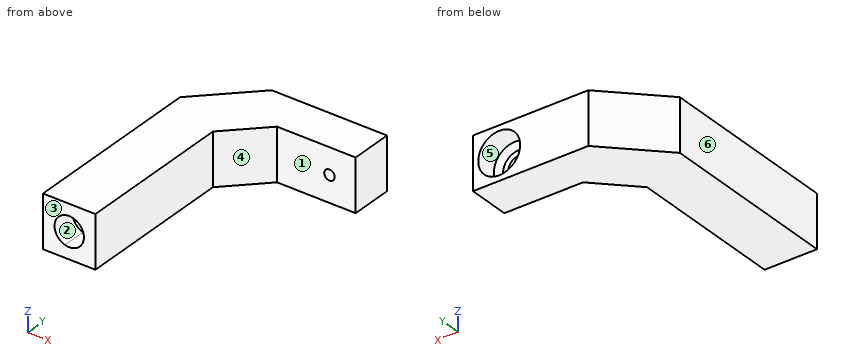
from build123d import *

# Parameters (mm, degrees)
PAD_DEPTH       = 10
CHAMFER_SIZE    = 10
POCKET_DEPTH    = 10.6
SKETCH002_R     = 2.8
POCKET001_DEPTH = 4.6
SKETCH003_R     = 1
POCKET002_DEPTH = 45.001
SKETCH004_R     = 4
POCKET003_DEPTH = 5
CHAMFER001_SIZE = 1
CHAMFER002_SIZE = 1


with BuildPart() as part:
    # Sketch → Pad (new body)
    with BuildSketch(Plane.XY):
        Polygon((22, 15), (-10, 15), (-10, -30), (0, -30), (0, 0), (7, 7), (22, 7), align=None)
    extrude(amount=PAD_DEPTH)

    # Chamfer
    chamfer_edges = [part.edges().sort_by_distance(p)[0] for p in [
        (-10, 15, 5),
    ]]
    chamfer(chamfer_edges, length=CHAMFER_SIZE)

    # Sketch001 → Pocket (cut)
    with BuildSketch(Plane.XZ.offset(30)):
        with BuildLine():
            ThreePointArc((-5.8, 2.316718), (-2.2, 5), (-5.8, 7.683282))
            Line((-5.8, 7.683282), (-5.8, 2.316718))
        make_face()
    extrude(amount=-POCKET_DEPTH, mode=Mode.SUBTRACT)

    # Sketch002 → Pocket001 (cut)
    with BuildSketch(Plane.XZ.offset(30)):
        with Locations((-5, 5)):
            Circle(SKETCH002_R)
    extrude(amount=-POCKET001_DEPTH, mode=Mode.SUBTRACT)

    # Sketch003 → Pocket002 (cut, through all)
    with BuildSketch(Plane(origin=(0, 15, 0), x_dir=(-1, 0, 0), z_dir=(0, 1, 0))):
        with Locations((-17, 5)):
            Circle(SKETCH003_R)
    extrude(amount=-POCKET002_DEPTH, mode=Mode.SUBTRACT)

    # Sketch004 → Pocket003 (cut)
    with BuildSketch(Plane(origin=(0, 15, 0), x_dir=(-1, 0, 0), z_dir=(0, 1, 0))):
        with Locations((-17, 5)):
            Circle(SKETCH004_R)
    extrude(amount=-POCKET003_DEPTH, mode=Mode.SUBTRACT)

    # Chamfer001
    chamfer001_edges = [part.edges().sort_by_distance(p)[0] for p in [
        (21, 10, 5),
    ]]
    chamfer(chamfer001_edges, length=CHAMFER001_SIZE)

    # Chamfer002
    chamfer002_edges = [part.edges().sort_by_distance(p)[0] for p in [
        (18, 10, 5),
    ]]
    chamfer(chamfer002_edges, length=CHAMFER002_SIZE)


solid = part.part
For this review, take the finished solid that the model builds, in its own axes (mm). Face numbers are marked on the shaded views. A direction names the side the tool comes from. Coordinates: 2 decimals unless noted, no trailing zeros. Write each loop counter-clockwise with the first axis right and the second up, starting at its lowest first coordinate (ties: lowest second). Pieces come first, ordered by that corner, then holes. Notation, with made-up numbers: (46.5, -37.5) -> (98.5, -37.5) arc R23 cw to (98.5, -14.5) -> close; hole circle Ø1 at (-27.75, 70). An arc over 180 degrees is marked (long way). Write each question's results on one line, items separated by ' | '. Start each with the question number.
1) For the marked faces 1, 2 and 3, list the 3-axis set-ups (+Z, -Z, +X, -X, +Y, -Y) from which the entire face can be reached by the end or side of a thin tool; tool diameter is ignored.
2) Consider section B-B (x = 17). Write out the cut boundary in (y, z).
3) Wall thickness on L1, parallel to X at y = -27.5, z = 5; L2, parallel to Z at x = 17, y = 12.5; L3, parallel to X at y = -22, z = 5: over which ranges is each line inside the solid? List them lowest first. Write a range as [from, to].
4) Consider section D-D (y = -5.5). Write out the cut boundary in (x, z).
5) Insertion check: pin 1 (12 mm diameter, centred on x = 18, y = 9, fed in from -Z); pin 2 (2.5 mm diameter, centred on x = 17, z = 5, fed in from +Y); pin 3 (1.1 mm diameter, centred on x = -4.5, z = 5, fed in from -Y); pin 4 (5 mm diameter, centred on x = 16.5, z = 6, fed in from +Y). Each pin has a flat end and moves straight along its axis. Give the tip position at first contact, or say it passes through.
6) Consider section A-A (z = 5). Write out the cut boundary in (x, y).
7) Consider section C-C (x = -5). Write out the cut boundary in (y, z).
8) The part is to be moulded in two halves that separate along X. For the marked faces 4, 5 and 6, say which applies: +X half, -X half, draft (parallel to the pull), parting line (faces both ways), or undercut.
Geometry says:
1) face 1: +Z, -Z, +X, -Y | face 2: -Y | face 3: +Z, -Z, +X, -X, -Y
2) outline: (7, 0) -> (15, 0) -> (15, 1) -> (11, 1) -> (10, 2) -> (10, 3) -> (9, 4) -> (7, 4) -> close; (7, 6) -> (9, 6) -> (10, 7) -> (10, 8) -> (11, 9) -> (15, 9) -> (15, 10) -> (7, 10) -> close
3) L1: [-10, -7.8], [-2.2, 0] | L2: [0, 1], [9, 10] | L3: [-10, -5.8], [-2.2, 0]
4) outline: (-10, 0) -> (0, 0) -> (0, 10) -> (-10, 10) -> close
5) pin 1: z = 0 | pin 2: y = 9.25 | pin 3: y = -19.4 | pin 4: y = 10.62
6) outline: (-10, -30) -> (-7.8, -30) -> (-7.8, -25.4) -> (-5.8, -25.4) -> (-5.8, -19.4) -> (-2.2, -19.4) -> (-2.2, -30) -> (0, -30) -> (0, 0) -> (7, 7) -> (16, 7) -> (16, 9) -> (15, 10) -> (14, 10) -> (13, 11) -> (13, 15) -> (0, 15) -> (-10, 5) -> close; (18, 7) -> (22, 7) -> (22, 15) -> (21, 15) -> (21, 11) -> (20, 10) -> (19, 10) -> (18, 9) -> close
7) outline: (-30, 0) -> (10, 0) -> (10, 10) -> (-30, 10) -> (-30, 7.8) -> (-19.4, 7.8) -> (-19.4, 2.2) -> (-30, 2.2) -> close
8) face 4: +X half | face 5: undercut | face 6: -X half
